Input: part model. Units: mm. Frame: model coordinates. A direction names the side the tool comes from. Coordinates: 2 decimals unless noted, no trailing zeros. Write each loop counter-clockwise with the first axis right and the second up, starting at its lowest first coordinate (ties: lowest second). Pieces come first, ordered by that corner, then holes. Notation, with made-up numbers: (-6.75, 33) -> (47.25, 33) arc R25 ccw to (47.25, 50) -> close; hole circle Ø5 at (73, 43.25). An arc over 180 degrees is marked (long way). Use one line per item in the form item = value. Start each with the question number.
(1) Cut plane B-B on y = 23. Return the cut outline in (x, z), plus the area to 3 significant figures.
(2) Cut plane C-C on y = 12. Return the cut outline in (x, z) (3 decimals), plus the area to 3 significant figures.
(3) Set-up query: faces 1 (the face through (3, -2, -1.298)), 2 (the face through (1.518, -2, -10)), 3 (the face through (3.38, 22.78, -5.17)), 4 (the face through (3, -2, -2.175)), 5 (the face through (3, -2, -10.77)). Return all of +Z, -Z, +X, -X, +Y, -Y with unobstructed straight access to the full face (end or side cutting, diameter ignored); none if empty.
(4) Cut plane A-A on z = -1.75. Return the cut outline in (x, y).
(5) Ray query, line 1 along Y through (x, z) = (2.75, -12); line 2 along Y through (x, z) = (3.25, -10.25); line 3 along Z through (x, y) = (2, 10.5). Return the intervals inside material, ascending.
(6) First-contact query: pin 1 (1.8 mm diameter, centred on x = 2.5, y = -2.5, fed in from -Z); pin 2 (4 mm diameter, centred on x = 2.5, y = -2.5, fed in from +Z); pin 3 (1.5 mm diameter, centred on y = 16.5, z = -3, fed in from +X). Flat tips, straight axial feed; report the tip coordinate or a pass-through.
```python
from build123d import *

# Parameters (mm, degrees)
SKETCH1_W           = 6.86
SKETCH1_H           = 12.7
BOSS_EXTRUDE1_DEPTH = 10
SKETCH2_W           = 3.547875369
SKETCH2_H           = 0.73404318
SKETCH2_H_2         = 0.876773798
SKETCH2_H_3         = 1.050089549
BOSS_EXTRUDE2_DEPTH = 4
SKETCH3_R           = 3.175
BOSS_EXTRUDE3_DEPTH = 8.89
SKETCH4_R           = 1.182295496
BOSS_EXTRUDE4_DEPTH = 8.89
FILLET1_R           = 1


with BuildPart() as part:
    # Sketch1 → Boss-Extrude1 (new body)
    with BuildSketch(Plane(origin=(0, 0, 0), x_dir=(1, 0, 0), z_dir=(0, 1, 0))):
        with Locations((3.43, 6.35)):
            Rectangle(SKETCH1_W, SKETCH1_H)
    extrude(amount=BOSS_EXTRUDE1_DEPTH)

    # Sketch2 → Boss-Extrude2 (add)
    with BuildSketch(Plane.XZ):
        with Locations((3.292366904, -6.538608317)):
            Rectangle(SKETCH2_W, SKETCH2_H)
        with Locations((3.292366904, -1.736742516)):
            Rectangle(SKETCH2_W, SKETCH2_H_2)
        with Locations((3.292366904, -10.244506871)):
            Rectangle(SKETCH2_W, SKETCH2_H_3)
    extrude(amount=BOSS_EXTRUDE2_DEPTH)

    # Sketch3 → Boss-Extrude3 (add)
    with BuildSketch(Plane(origin=(0, 10, 0), x_dir=(1, 0, 0), z_dir=(0, 1, 0))):
        with Locations(Location((3.43, 6.35, 0), (0, 0, 90))):
            Circle(SKETCH3_R)
    extrude(amount=BOSS_EXTRUDE3_DEPTH)

    # Sketch4 → Boss-Extrude4 (add)
    with BuildSketch(Plane(origin=(0, 18.89, 0), x_dir=(1, 0, 0), z_dir=(0, 1, 0))):
        with Locations(Location((3.43, 6.35, 0), (0, 0, 90))):
            Circle(SKETCH4_R)
    extrude(amount=BOSS_EXTRUDE4_DEPTH)

    # Fillet1
    fillet1_edges = [part.edges().sort_by_distance(p)[0] for p in [
        (3.43, 27.78, -5.167704504),
    ]]
    fillet(fillet1_edges, radius=FILLET1_R)


solid = part.part
```
Values:
q1.outline = circle Ø2.36 at (3.43, -6.35)
q1.area = 4.39 mm2
q2.outline = circle Ø6.35 at (3.43, -6.35)
q2.area = 31.7 mm2
q3.face_1 = +Z, +X, -X, -Y
q3.face_2 = +Z, -Z, -X, -Y
q3.face_3 = +Y
q3.face_4 = +X, -X, -Y
q3.face_5 = -Z, +X, -X, -Y
q4.outline = (0, 0) -> (1.52, 0) -> (1.52, -4) -> (5.07, -4) -> (5.07, 0) -> (6.86, 0) -> (6.86, 10) -> (0, 10) -> close
q5.line_1 = 0 to 10
q5.line_2 = -4 to 10
q5.line_3 = -9.18 to -3.52
q6.pin_1 = -10.77
q6.pin_2 = -1.3
q6.pin_3 = 5.25
